Answer from the drawing. Dimensions are ordinates in mm from the lowest x, y and z of the part. A direction names the side the tool comes from. Give positions to 0.01 mm unless a question says otherwise; leave off trailing zeros. Loops run counter-clockwise (first coordinate to the right, second up) from the corner with the lowest first, then second, coordinate; pieces in that order, holes last.
Item 1: The mould has two halves that part along X. Classify the marked faces 6, 7, 8 and 9: pulls with the +X half, pulls with the -X half, needs draft (parallel to the pull), parting line crosses it, or undercut.
Item 2: Section B-B, the plane x = 25 is taken. Give the vertices of the cut face in (y, z), and give its area (3 significant figures).
Item 3: Section C-C, the plane y = 10 is taken. Give the vertices of the cut face in (x, z), and give its area (3 significant figures).
Item 4: Each of these flat-tipped pins is pushed along its axis until it touches: pin 1 Ø2.5 at (y, z) = (2, 13) entering from -X; pin 2 Ø7.5 at (x, z) = (24.5, 9.5) entering from +Y; pin 3 Ø4 at (x, y) = (40.5, 11) entering from +Z; pin 4 Ø10 at (x, y) = (44, 11) entering from -Z. Where does it stop, or does it pass through?
Item 5: Section A-A, the plane z = 2.5 is taken. Give the vertices of the cut face in (x, y).
Item 6: Section D-D, the plane y = 3.5 is taken. Give the vertices of the cut face in (x, z).
Item 7: Consider line 1 along Y through (x, z) = (16.5, 1.1); line 2 along Y through (x, z) = (25, 1.3); line 3 along Z through (x, y) = (3.5, 5.5). Determine where each line is inside the solid, lowest interval first.
Item 8: A tool of negligible diameter and unlimited length cuts with its end or side. For the marked faces 1, 2, 3, 4 and 5, from which of +Z, -Z, +X, -X, +Y, -Y can it reach the whole face along a straight path? Write none if from no direction.
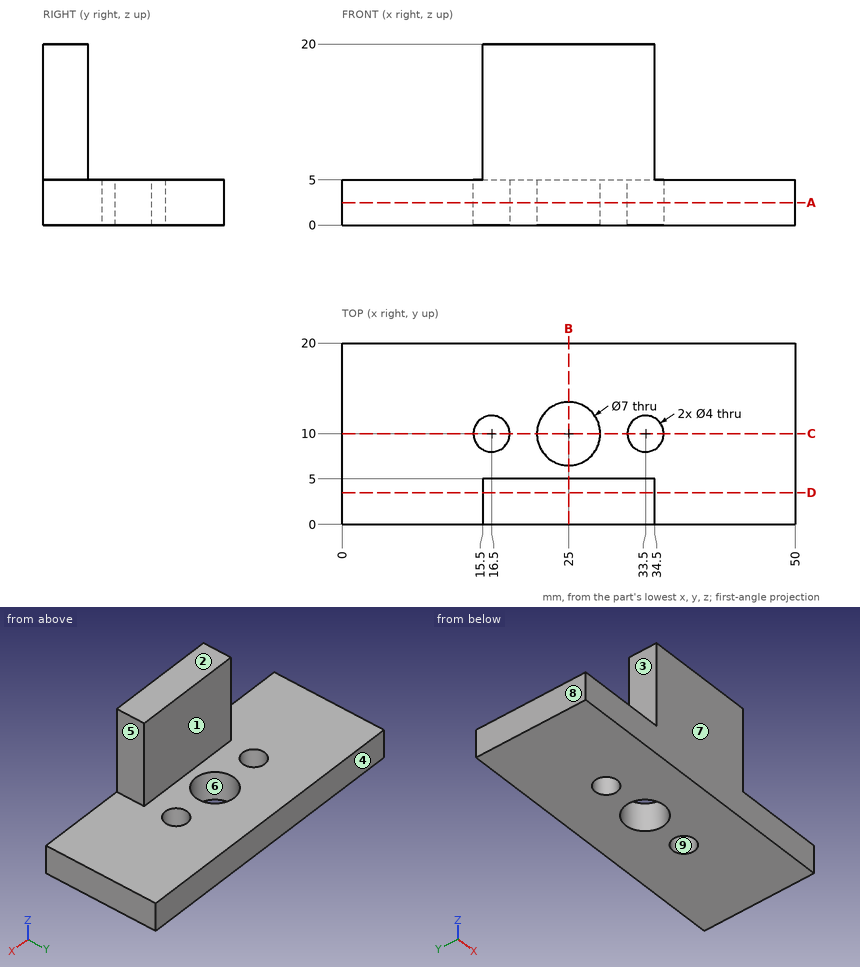
Worked answers:
1. face 6: undercut
1. face 7: needs draft
1. face 8: pulls with the -X half
1. face 9: undercut
2. outline: (0, 0) - (6.5, 0) - (6.5, 5) - (5, 5) - (5, 20) - (0, 20) - close; (13.5, 0) - (20, 0) - (20, 5) - (13.5, 5) - close
2. area: 140 mm2
3. outline: (0, 0) - (14.5, 0) - (14.5, 5) - (0, 5) - close; (18.5, 0) - (21.5, 0) - (21.5, 5) - (18.5, 5) - close; (28.5, 0) - (31.5, 0) - (31.5, 5) - (28.5, 5) - close; (35.5, 0) - (50, 0) - (50, 5) - (35.5, 5) - close
3. area: 175 mm2
4. pin 1: stops at x = 15.5
4. pin 2: stops at y = 5
4. pin 3: stops at z = 5
4. pin 4: stops at z = 0
5. outline: (0, 0) - (50, 0) - (50, 20) - (0, 20) - close; hole circle Ø4 at (16.5, 10); hole circle Ø7 at (25, 10); hole circle Ø4 at (33.5, 10)
6. outline: (0, 0) - (50, 0) - (50, 5) - (34.5, 5) - (34.5, 20) - (15.5, 20) - (15.5, 5) - (0, 5) - close
7. line 1: y = 0 to 8, 12 to 20
7. line 2: y = 0 to 6.5, 13.5 to 20
7. line 3: z = 0 to 5
8. face 1: +Z, +X, -X, +Y
8. face 2: +Z, +X, -X, +Y, -Y
8. face 3: +Z, -X, +Y, -Y
8. face 4: +Z, -Z, +X, -X, +Y
8. face 5: +Z, +X, +Y, -Y
